```python
from build123d import *

# Parameters (mm, degrees)
CUT_EXTRUDE1_DEPTH = 8


with BuildPart() as part:
    # Sketch1 → Revolve1 (revolve)
    with BuildSketch(Plane.XY):
        with BuildLine():
            Line((-9.946660926, -3.531651516), (-9.946660926, -12.5))
            Line((-9.946660926, -12.5), (-4.946660926, -12.5))
            Line((-4.946660926, -12.5), (-4.946660926, -12.3))
            Line((-4.946660926, -12.3), (6.053339074, -12.3))
            Line((6.053339074, -12.3), (6.053339074, -12.5))
            Line((6.053339074, -12.5), (11.053339074, -12.5))
            Line((11.053339074, -12.5), (11.053339074, -11.2))
            ThreePointArc((11.053339074, -11.2), (11.346232293, -11.907106781), (12.053339074, -12.2))
            Line((12.053339074, -12.2), (42.053339074, -12.2))
            Line((42.053339074, -12.2), (42.053339074, -3.25))
            Line((42.053339074, -3.25), (43.853339074, -3.25))
            ThreePointArc((43.853339074, -3.25), (43.99476043, -3.191421356), (44.053339074, -3.05))
            Line((44.053339074, -3.05), (44.053339074, 0))
            Line((44.053339074, 0), (-21.446660926, 0))
            Line((-21.446660926, 0), (-21.446660926, -1.5))
            Line((-21.446660926, -1.5), (-20.946660926, -2))
            Line((-20.946660926, -2), (-12.446660926, -2))
            Line((-12.446660926, -2), (-12.446660926, -3.531651516))
            Line((-12.446660926, -3.531651516), (-9.946660926, -3.531651516))
        make_face()
    revolve(axis=Axis((-21.446660926, 0, 0), (1, 0, 0)))

    # Sketch2 → Cut-Extrude1 (cut)
    with BuildSketch(Plane.ZY.offset(21.446660926)):
        with BuildLine():
            Line((-1.322875656, 1.5), (1.322875656, 1.5))
            ThreePointArc((1.322875656, 1.5), (0, 2), (-1.322875656, 1.5))
        make_face()
    extrude(amount=-CUT_EXTRUDE1_DEPTH, mode=Mode.SUBTRACT)


solid = part.part
```
Here's how the part is built. I have some questions about the finished solid (model axes, mm). A direction names the side the tool comes from. Coordinates: 2 decimals unless noted, no trailing zeros. Write each loop counter-clockwise with the first axis right and the second up, starting at its lowest first coordinate (ties: lowest second). Pieces come first, ordered by that corner, then holes. Notation, with made-up numbers: (64.5, 24) - (98.5, 24) arc R24 cw to (98.5, 47) - close; hole circle Ø1 at (48, 44.5). An arc over 180 degrees is marked (long way). One line per item, written item: value.
1) I need wall thicknesses on line 1 along X through (y, z) = (-7.25, 5); line 2 along Y through (x, z) = (10.5, -2.75); line 3 along X through (y, z) = (-3, -1.5). Which ranges of each line are inside material? Lowest first, please.
Model answer:
line 1: x = -9.95 to 42.05
line 2: y = -12.19 to 12.19
line 3: x = -12.45 to 42.05
2) Suppose I cut it at C-C on x = -3. Write out the boundary of the cut face in (y, z).
Model answer:
outline: circle Ø24.6 at (0, 0)
3) I'm going to push flat-ended pins straight in: P1, Ø1.5, axis at y = 2.5, z = 6.5, coming from the +X side; P2, Ø6, axis at x = 31.5, y = -4.5, coming from the -Z side; P3, Ø3, axis at x = 22, y = 4.5, coming from the -Z side. Where does each tip first touch, or does it pass through?
Model answer:
P1: stops at x = 42.05
P2: stops at z = -12.11
P3: stops at z = -11.83
4) Suppose I cut it at B-B on x = 19. Write out the boundary of the cut face in (y, z), and give its area (3 significant figures).
Model answer:
outline: circle Ø24.4 at (0, 0)
area: 468 mm²
5) On a 3-axis mill with a long thin cutter (end or side, diameter ignored), from which of +Z, -Z, +X, -X, +Y, -Y can I reach the whole of each face in a straight line? I mean faces 1 (the cylindrical face through (8.588, -11.923, -3.755)), 2 (the cylindrical face through (0.6, 2.7, 12)), 3 (the flat face through (-18, 1.5, 0)), 4 (the cylindrical face through (-16.637, -1.908, -0.601)), 5 (the flat face through (42.053, -3, 3)). Say none if no direction works.
Model answer:
face 1: +X, -X
face 2: none
face 3: +Z, -Z, -X, +Y
face 4: -X
face 5: +X
